Read the model definition and answer for the solid it produces. Units are mm, in the model's axes. A direction names the side the tool comes from. Give positions to 0.01 mm unless a question says otherwise; leave off trailing zeros. Write each loop counter-clockwise with the first axis right and the second up, starting at its lowest first coordinate (ties: lowest second). Pieces come first, ordered by that corner, then holes. Notation, with made-up numbers: M 77.25,-20 L 118.25,-20 A23 ccw 118.25,19 Z; hole C 69.25,6 d6. An arc over 180 degrees is marked long. Write each question's results on one line, items separated by ' | '. Start each with the question number.
Autodesk Inventor part; units mm, degrees
ref_plane "YZ Plane" through (0, 0, 0) normal (1, 0, 0) x (0, 1, 0)
ref_plane "XZ Plane" through (0, 0, 0) normal (0, 1, 0) x (-1, 0, 0)
ref_plane "XY Plane" through (0, 0, 0) normal (0, 0, 1) x (1, 0, 0)
sketch "スケッチ1" plane through (0, 0, 0) normal (0, 0, 1) x (1, 0, 0)
  line L0 (7.5, -7.5) -> (-7.5, -7.5)
  line L1 (-7.5, -7.5) -> (-7.5, 7.5)
  line L2 (-7.5, 7.5) -> (7.5, 7.5)
  line L3 (7.5, 7.5) -> (7.5, -7.5)
  line L4 (7.5, -7.5) -> (-7.5, 7.5) construction
  line L5 (-7.5, -7.5) -> (7.5, 7.5) construction
  line L6 (6.5, 6.5) -> (-6.5, 6.5)
  line L7 (-6.5, 6.5) -> (-6.5, -6.5)
  line L8 (-6.5, -6.5) -> (6.5, -6.5)
  line L9 (6.5, -6.5) -> (6.5, 6.5)
  point P0 (0, 0)
  dimension "d0" = 15
  dimension "d1" = 15
  dimension "d2" = 1
extrude "押し出し1" add sketch "スケッチ1" along normal blind 390
sketch "スケッチ2" plane through (7.5, -7.5, 0) normal (1, 0, 0) x (0, 0, -1)
  line L0 (0, 0) -> (0, 15)
  line L1 (0, 15) -> (-390, 15)
  line L2 (-390, 0) -> (-390, 15)
  line L3 (0, 0) -> (-390, 0)
  line L4 (0, 7.5) -> (-390, 7.5)
  point P0 (-380, 7.5)
  point P1 (-370, 7.5)
  point P2 (-10, 7.5)
  point P3 (-20, 7.5)
  point P4 (-360, 7.5)
  point P5 (-30, 7.5)
  dimension "d5" = 10
  dimension "d6" = 10
  dimension "d7" = 10
  dimension "d8" = 10
  dimension "d27" = 10
  dimension "d28" = 10
hole "穴1" at (7.5, 0, 380) at (7.5, 0, 370) at (7.5, 0, 10) at (7.5, 0, 20) at (7.5, 0, 30) at (7.5, 0, 360) direction (-1, 0, 0) diameter 3.3 end through all
sketch "スケッチ3" plane through (-7.5, -7.5, 0) normal (0, -1, 0) x (1, 0, 0)
  line L0 (0, 0) -> (15, 0)
  line L1 (15, 0) -> (15, 390)
  line L2 (0, 390) -> (15, 390)
  line L3 (0, 0) -> (0, 390)
  line L4 (7.5, 0) -> (7.5, 390)
  point P0 (7.5, 360)
  point P1 (7.5, 350)
  point P2 (7.5, 40)
  point P3 (7.5, 30)
  dimension "d16" = 10
  dimension "d17" = 10
  dimension "d18" = 30
  dimension "d19" = 30
hole "穴2" at (0, -7.5, 360) at (0, -7.5, 350) at (0, -7.5, 40) at (0, -7.5, 30) direction (0, 1, 0) diameter 3.2 end through all
properties part number "light_kaku_connect"
Item 1: Determine the mould class of faces 1 (the flat face through (-6.5, 0, 192)), 2 (the flat face through (7.5, 0, 192)), 3 (the flat face through (0, 7.5, 192)) for opening direction Y: +Y half, -Y half, draft (parallel to the pull), parting line (faces both ways), or undercut.
Item 2: Section A-A, the plane x = -4 is taken. Determine the outline of the cut face in (y, z).
Item 3: Straight lines are drawn through the part: line 1 (Z direction, x = 0, y = 7.05); line 2 (X direction, y = -7.05, z = 30); line 3 (X direction, y = -0.75, z = 317). For each, find the intervals that lie inside material, in ascending order.
Item 4: Section B-B, the plane z = 302 is taken. Determine the outline of the cut face in (x, y), then the cut area to 3 significant figures.
Item 5: For faces 4 (the flat face through (-7, 0, 390)), 5 (the flat face through (6.5, 0, 192)), determine the directions among +Z, -Z, +X, -X, +Y, -Y from which every point of the face is accessible in a straight line to the end or side of a thin tool.
Item 6: Given P1, Ø2, axis at y = 0, z = 30, coming from the +X side, flat-ended and moving along its own axis, determine where the tip first touches the part or whether it passes through.
Worked out:
1) face 1: undercut | face 2: draft | face 3: +Y half
2) outline: M -7.5,0 L -6.5,0 L -6.5,390 L -7.5,390 Z; M 6.5,0 L 7.5,0 L 7.5,390 L 6.5,390 Z
3) line 1: z = 0 to 28.4, 31.6 to 38.4, 41.6 to 348.4, 351.6 to 358.4, 361.6 to 390 | line 2: x = -7.5 to -1.6, 1.6 to 7.5 | line 3: x = -7.5 to -6.5, 6.5 to 7.5
4) outline: M -7.5,-7.5 L 7.5,-7.5 L 7.5,7.5 L -7.5,7.5 Z; hole M -6.5,-6.5 L 6.5,-6.5 L 6.5,6.5 L -6.5,6.5 Z | area: 56.0 mm²
5) face 4: +Z, +X, -X, +Y, -Y | face 5: +Z, -Z
6) P1: passes through
